```python
from build123d import *

# Parameters (mm, degrees)
SKETCH1_W           = 40
SKETCH1_H           = 40
SKETCH1_R           = 1.6
SKETCH1_R_2         = 6.25
BOSS_EXTRUDE1_DEPTH = 2
SKETCH2_W           = 40
SKETCH2_H           = 25
BOSS_EXTRUDE2_DEPTH = 2
SKETCH3_W           = 8
SKETCH3_H           = 23
BOSS_EXTRUDE3_DEPTH = 15
CUT_EXTRUDE1_DEPTH  = 15
SKETCH5_R           = 1.6
CUT_EXTRUDE2_DEPTH  = 15
BOSS_EXTRUDE4_START = 2
SKETCH8_R           = 1.6
SKETCH8_R_2         = 6.25
BOSS_EXTRUDE4_DEPTH = 2
CUT_EXTRUDE6_START  = -2
SKETCH9_R           = 6.25
SKETCH9_R_2         = 1.6
CUT_EXTRUDE6_DEPTH  = 2
CUT_EXTRUDE5_START  = -10
SKETCH7_W           = 8
SKETCH7_H           = 5.7
CUT_EXTRUDE5_DEPTH  = 3
SKETCH10_W          = 15
SKETCH10_H          = 27
SKETCH10_R          = 3.25
BOSS_EXTRUDE5_DEPTH = 2
FILLET2_START       = -1
FILLET2_DEPTH       = 26
FILLET3_R           = 1
FILLET4_R           = 3


with BuildPart() as part:
    # Sketch1 → Boss-Extrude1 (new body)
    with BuildSketch(Plane.XY):
        Rectangle(SKETCH1_W, SKETCH1_H)
        with Locations((-15.5, 0)):
            Circle(SKETCH1_R, mode=Mode.SUBTRACT)
        with Locations((7.75, 13.423393759)):
            Circle(SKETCH1_R, mode=Mode.SUBTRACT)
        with Locations((7.75, -13.423393759)):
            Circle(SKETCH1_R, mode=Mode.SUBTRACT)
        with Locations((0, 7)):
            Circle(SKETCH1_R_2, mode=Mode.SUBTRACT)
    extrude(amount=BOSS_EXTRUDE1_DEPTH)

    # Sketch2 → Boss-Extrude2 (add)
    with BuildSketch(Plane(origin=(0, 20, 0), x_dir=(1, 0, 0), z_dir=(0, 1, 0))):
        with Locations((0, -12.5)):
            Rectangle(SKETCH2_W, SKETCH2_H)
    extrude(amount=BOSS_EXTRUDE2_DEPTH)

    # Sketch3 → Boss-Extrude3 (add)
    with BuildSketch(Plane.XZ.offset(-20)):
        with Locations((-16, 13.5)):
            Rectangle(SKETCH3_W, SKETCH3_H)
        with Locations((16, 13.5)):
            Rectangle(SKETCH3_W, SKETCH3_H)
    extrude(amount=BOSS_EXTRUDE3_DEPTH)

    # Sketch4 → Cut-Extrude1 (cut)
    with BuildSketch(Plane.XY.offset(2)):
        with BuildLine():
            ThreePointArc((3.6e-08, -20), (-14.142135611, -14.142135636), (-20, 0))
            Line((-20, 0), (-20, -20))
            Line((-20, -20), (3.6e-08, -20))
        make_face()
        with BuildLine():
            ThreePointArc((20, 0), (14.142135636, -14.142135611), (3.6e-08, -20))
            Line((3.6e-08, -20), (20, -20))
            Line((20, -20), (20, 0))
        make_face()
    extrude(amount=-CUT_EXTRUDE1_DEPTH, mode=Mode.SUBTRACT)

    # Sketch5 → Cut-Extrude2 (cut)
    with BuildSketch(Plane.XZ.offset(-5)):
        with Locations(Location((-16, 7.75, 0), (0, 0, 270))):
            Circle(SKETCH5_R)
        with Locations(Location((-16, 19.25, 0), (0, 0, 270))):
            Circle(SKETCH5_R)
        with Locations(Location((16, 7.75, 0), (0, 0, 90))):
            Circle(SKETCH5_R)
        with Locations(Location((16, 19.25, 0), (0, 0, 90))):
            Circle(SKETCH5_R)
    extrude(amount=-CUT_EXTRUDE2_DEPTH, mode=Mode.SUBTRACT)

    # Sketch8 → Boss-Extrude4 (add)
    with BuildSketch(Plane(origin=(0, 0, 0), x_dir=(-1, 0, 0), z_dir=(0, 0, -1)).offset(BOSS_EXTRUDE4_START)):
        with BuildLine():
            Line((-20, 22), (-20, 0))
            ThreePointArc((-20, 0), (0, -20), (20, 0))
            Line((20, 0), (20, 22))
            Line((20, 22), (-20, 22))
        make_face()
        with Locations((-7.75, 13.423393759)):
            Circle(SKETCH8_R, mode=Mode.SUBTRACT)
        with Locations((0, 7)):
            Circle(SKETCH8_R_2, mode=Mode.SUBTRACT)
        with Locations((15.5, 0)):
            Circle(SKETCH8_R, mode=Mode.SUBTRACT)
        with Locations((-7.75, -13.423393759)):
            Circle(SKETCH8_R, mode=Mode.SUBTRACT)
    extrude(amount=-BOSS_EXTRUDE4_DEPTH)

    # Sketch9 → Cut-Extrude6 (cut)
    with BuildSketch(Plane.XY.offset(2).offset(CUT_EXTRUDE6_START)):
        with BuildLine():
            Line((20, 0), (20, 5))
            Line((20, 5), (12, 5))
            Line((12, 5), (12, 20))
            Line((12, 20), (-12, 20))
            Line((-12, 20), (-12, 5))
            Line((-12, 5), (-20, 5))
            Line((-20, 5), (-20, 0))
            ThreePointArc((-20, 0), (0, -20), (20, 0))
        make_face()
        with Locations(Location((0, 7, 0), (0, 0, 180))):
            Circle(SKETCH9_R, mode=Mode.SUBTRACT)
        with Locations(Location((7.75, 13.423393759, 0), (0, 0, 180))):
            Circle(SKETCH9_R_2, mode=Mode.SUBTRACT)
        with Locations(Location((-15.5, 0, 0), (0, 0, 180))):
            Circle(SKETCH9_R_2, mode=Mode.SUBTRACT)
        with Locations(Location((7.75, -13.423393759, 0), (0, 0, 180))):
            Circle(SKETCH9_R_2, mode=Mode.SUBTRACT)
    extrude(amount=CUT_EXTRUDE6_DEPTH, mode=Mode.SUBTRACT)

    # Sketch7 → Cut-Extrude5 (cut)
    with BuildSketch(Plane.XZ.offset(-5).offset(CUT_EXTRUDE5_START)):
        with Locations((-16, 19.25)):
            Rectangle(SKETCH7_W, SKETCH7_H)
        with Locations((16, 19.25)):
            Rectangle(SKETCH7_W, SKETCH7_H)
        with Locations((16, 7.75)):
            Rectangle(SKETCH7_W, SKETCH7_H)
        with Locations((-16, 7.75)):
            Rectangle(SKETCH7_W, SKETCH7_H)
    extrude(amount=CUT_EXTRUDE5_DEPTH, mode=Mode.SUBTRACT)

    # Sketch10 → Boss-Extrude5 (add)
    # profile 1 of 2: a face of its own
    with BuildSketch(Plane.XZ.offset(-20)):
        with Locations((-27.5, 11.5)):
            Rectangle(SKETCH10_W, SKETCH10_H)
        with Locations(Location((-27.5, 11.5, 0), (0, 0, 270))):
            Circle(SKETCH10_R, mode=Mode.SUBTRACT)
    # profile 2 of 2: a face of its own
    with BuildSketch(Plane.XZ.offset(-20)):
        with Locations((27.5, 11.5)):
            Rectangle(SKETCH10_W, SKETCH10_H)
        with Locations(Location((27.5, 11.5, 0), (0, 0, 270))):
            Circle(SKETCH10_R, mode=Mode.SUBTRACT)
    extrude(amount=-BOSS_EXTRUDE5_DEPTH)

    # Fillet2: read off the stored shape, not the designer's step
    # Fillet2 outline → Fillet2 (add)
    with BuildSketch(Plane.XY.offset(FILLET2_START)):
        with BuildLine():
            ThreePointArc((-12, 15), (-10.535533906, 18.535533906), (-7, 20))
            Line((-7, 20), (-12, 20))
            Line((-12, 20), (-12, 15))
        make_face()
        with BuildLine():
            ThreePointArc((7, 20), (10.535533906, 18.535533906), (12, 15))
            Line((12, 15), (12, 20))
            Line((12, 20), (7, 20))
        make_face()
    extrude(amount=FILLET2_DEPTH)

    # Fillet3
    fillet3_edges = [part.edges().sort_by_distance(p)[0] for p in [
        (-20, 20, 11.5),
        (20, 20, 11.5),
    ]]
    fillet(fillet3_edges, radius=FILLET3_R)

    # Fillet4
    fillet4_edges = [part.edges().sort_by_distance(p)[0] for p in [
        (-35, 21, -2),
        (-35, 21, 25),
        (35, 21, 25),
        (35, 21, -2),
    ]]
    fillet(fillet4_edges, radius=FILLET4_R)


solid = part.part
```
For this review, take the finished solid that the model builds, in its own axes (mm). A direction names the side the tool comes from. Round coordinates to 2 decimals unless told otherwise and drop trailing zeros. Order: outer loops, then holes, each group sorted by start corner. A loop starts at its lowest first (then second) coordinate and runs counter-clockwise, first axis right, second up. Notation, with made-up numbers: (-37.75, 75) -> (-3.75, 75) arc R32 ccw to (-3.75, 109) -> close; hole circle Ø7 at (18.25, 58). An arc over 180 degrees is marked (long way). Use a Markdown table: item, result.
Item 1: Take a section at A-A (x = 27.5). State the section outline as (y, z) points, plus the area to 3 significant figures.
Resolved:
| item | result |
|---|---|
| outline | (20, -2) -> (22, -2) -> (22, 8.25) -> (20, 8.25) -> close; (20, 14.75) -> (22, 14.75) -> (22, 25) -> (20, 25) -> close |
| area | 41.0 mm² |
Item 2: For line 1 along Z through (x, y) = (16, 17.1); line 2 along X through (y, z) = (20.8, 11.5); line 3 along X through (y, z) = (6.75, 19.25), list the stretches that pass through material, from the lowest coordinate up. Write a range as [from, to].
Resolved:
| item | result |
|---|---|
| line 1 | z = [-2, 6.15], [9.35, 17.65], [20.85, 25] |
| line 2 | x = [-35, -30.75], [-24.25, 24.25], [30.75, 35] |
| line 3 | x = [-20, -17.6], [-14.4, -12], [12, 14.4], [17.6, 20] |
Item 3: Take a section at C-C (y = 7). State the section outline as (x, z) points.
Resolved:
| item | result |
|---|---|
| outline | (-20, -2) -> (-6.25, -2) -> (-6.25, 0) -> (-12, 0) -> (-12, 25) -> (-20, 25) -> close; (6.25, -2) -> (20, -2) -> (20, 25) -> (12, 25) -> (12, 0) -> (6.25, 0) -> close; hole circle Ø3.2 at (-16, 7.75); hole circle Ø3.2 at (-16, 19.25); hole circle Ø3.2 at (16, 7.75); hole circle Ø3.2 at (16, 19.25) |
Item 4: Take a section at D-D (z = 3.5). State the section outline as (x, y) points.
Resolved:
| item | result |
|---|---|
| outline | (-35, 20) -> (-21, 20) arc R1 cw to (-20, 19) -> (-20, 5) -> (-12, 5) -> (-12, 15) arc R5 cw to (-7, 20) -> (7, 20) arc R5 cw to (12, 15) -> (12, 5) -> (20, 5) -> (20, 19) arc R1 cw to (21, 20) -> (35, 20) -> (35, 22) -> (-35, 22) -> close |
Item 5: Take a section at B-B (z = 11.5). State the section outline as (x, y) points.
Resolved:
| item | result |
|---|---|
| outline | (-35, 20) -> (-30.75, 20) -> (-30.75, 22) -> (-35, 22) -> close; (-24.25, 20) -> (-21, 20) arc R1 cw to (-20, 19) -> (-20, 5) -> (-12, 5) -> (-12, 15) arc R5 cw to (-7, 20) -> (7, 20) arc R5 cw to (12, 15) -> (12, 5) -> (20, 5) -> (20, 19) arc R1 cw to (21, 20) -> (24.25, 20) -> (24.25, 22) -> (-24.25, 22) -> close; (30.75, 20) -> (35, 20) -> (35, 22) -> (30.75, 22) -> close |
Item 6: Machinability: for faces 1 (the flat face through (20, 12, 11)), 2 (the cylindrical face through (10, 19, 12)), 3 (the cylindrical face through (14.92, 8.45, 6.57)), 4 (the flat face through (16, 14, 16.4)), 5 (the flat face through (-20, 11, 11)), which of the approach directions +Z, -Z, +X, -X, +Y, -Y give a long, thin tool a straight path to every point of the face, cutting with its end or side? Answer none if there is none.
Resolved:
| item | result |
|---|---|
| face 1 | +Z, -Z, +X, -Y |
| face 2 | +Z, -Y |
| face 3 | -Y |
| face 4 | +X, -X |
| face 5 | +Z, -Z, -X, -Y |
Item 7: For pin 1 (10 mm diameter, centred on x = -16, z = 8, fed in from -Y); pin 2 (11 mm diameter, centred on x = -30, z = 17, fed in from -Y); pin 3 (3 mm diameter, centred on x = -15.5, y = 0, fed in from -Z); pin 4 (1 mm diameter, centred on y = 11.5, z = 21.5, fed in from -X), all flat-tipped, find the tip position at first contact; note any pin that passes through.
Resolved:
| item | result |
|---|---|
| pin 1 | stops at y = 5 |
| pin 2 | stops at y = 20 |
| pin 3 | passes through |
| pin 4 | stops at x = -20 |
Item 8: Draft analysis for pull direction X (two halves, no side actions). For faces 6 (the cylindrical face through (-14.92, 8.45, 20.43)), 7 (the flat face through (16, 20, 19)), 8 (the cylindrical face through (-34.14, 21.01, -1.1)), 9 (the flat face through (-18, 15, 8)), state which applies: +X half, -X half, draft (parallel to the pull), parting line (faces both ways), or undercut.
Resolved:
| item | result |
|---|---|
| face 6 | undercut |
| face 7 | undercut |
| face 8 | -X half |
| face 9 | draft |
